```python
from build123d import *

# Parameters (mm, degrees)
BOSS_EXTRUDE1_DEPTH = 5
SKETCH2_R           = 2.5
BOSS_EXTRUDE2_DEPTH = 5
BOSS_EXTRUDE3_START = -2.644184
BOSS_EXTRUDE3_DEPTH = 127.644184


with BuildPart() as part:
    # Sketch1 → Boss-Extrude1 (new body)
    with BuildSketch(Plane(origin=(0, 0, 0), x_dir=(1, 0, 0), z_dir=(0, 1, 0))):
        with BuildLine():
            ThreePointArc((-22.5, 0), (0, -22.5), (22.5, 0))
            ThreePointArc((22.5, 0), (28.11402228, 25.340983158), (43.905514247, 45.939804848))
            ThreePointArc((43.905514247, 45.939804848), (54.788632448, 47.238126581), (60.325213459, 37.779047778))
            ThreePointArc((60.325213459, 37.779047778), (48.023832429, 20.66372887), (43.868302884, 0))
            ThreePointArc((43.868302884, 0), (0, -43.868302884), (-43.868302884, 0))
            ThreePointArc((-43.868302884, 0), (-48.023832429, 20.66372887), (-60.325213459, 37.779047778))
            ThreePointArc((-60.325213459, 37.779047778), (-54.788632448, 47.238126581), (-43.905514247, 45.939804848))
            ThreePointArc((-43.905514247, 45.939804848), (-28.11402228, 25.340983158), (-22.5, 0))
        make_face()
    extrude(amount=BOSS_EXTRUDE1_DEPTH)

    # Sketch2 → Boss-Extrude2 (add)
    with BuildSketch(Plane(origin=(0, 5, 0), x_dir=(1, 0, 0), z_dir=(0, 1, 0))):
        with Locations((28.779245994, -28.779245994)):
            Circle(SKETCH2_R)
        with Locations((-28.779245994, -28.779245994)):
            Circle(SKETCH2_R)
    extrude(amount=BOSS_EXTRUDE2_DEPTH)

    # Sketch4 → Boss-Extrude3 (add)
    with BuildSketch(Plane(origin=(0, 5, 43.868302884), x_dir=(1, 0, 0), z_dir=(0, 0, 1)).offset(BOSS_EXTRUDE3_START)):
        with BuildLine():
            Line((12.5, -5), (-12.5, -5))
            ThreePointArc((-12.5, -5), (-15, -2.5), (-12.5, 0))
            Line((-12.5, 0), (12.5, 0))
            ThreePointArc((12.5, 0), (15, -2.5), (12.5, -5))
        make_face()
    extrude(amount=BOSS_EXTRUDE3_DEPTH)


solid = part.part
```
Build history of the part. All positions in model axes, mm. A direction names the side the tool comes from. Round coordinates to 2 decimals unless told otherwise and drop trailing zeros. Write each loop counter-clockwise with the first axis right and the second up, starting at its lowest first coordinate (ties: lowest second). Pieces come first, ordered by that corner, then holes. Notation, with made-up numbers: (62.25, -38) -> (108.25, -38) arc R16 cw to (108.25, -30) -> close; hole circle Ø6 at (-10.5, 47.25). An arc over 180 degrees is marked (long way). Put each result on its own line as item: value.
Item 1: Two-plate mould, pull along X, no slides. Class faces 1 (the face through (15, 2.6, 104.2)), 2 (the face through (-28.27, 2.46, -25.67)), 3 (the face through (29, 10, 29)), 4 (the face through (-0.495, 2.465, 22.495)): pulls with the +X half, pulls with the -X half, needs draft (parallel to the pull), parting line crosses it, or undercut.
Here are the results:
face 1: pulls with the +X half
face 2: undercut
face 3: needs draft
face 4: undercut
Item 2: Tool access for faces 5 (the face through (27.96, 2.46, -25.01)), 6 (the face through (-15, 2.4, 104.2)), 7 (the face through (30.12, 7.46, 26.67)): list every direction of +Z, -Z, +X, -X, +Y, -Y with a clear straight run to the whole face (end or side of a thin tool).
Here are the results:
face 5: -Z, +Y, -Y
face 6: +Z, -X
face 7: +Y
Item 3: Slice it at A-A, the plane z = -22.5. Give the cut face in (x, y).
Here are the results:
outline: (-48.87, 0) -> (-26.88, 0) -> (-26.88, 5) -> (-48.87, 5) -> close; (26.88, 0) -> (48.87, 0) -> (48.87, 5) -> (26.88, 5) -> close
Item 4: Slice it at B-B, the plane y = 2.5. Give the cut face in (x, z), plus the area to 3 significant figures.
Here are the results:
outline: (-60.33, -37.78) arc R10 ccw to (-43.91, -45.94) arc R60 ccw to (-22.5, 0) arc R22.5 cw to (22.5, 0) arc R60 ccw to (43.91, -45.94) arc R10 ccw to (60.33, -37.78) arc R50 cw to (43.87, 0) arc R43.87 ccw to (15, 41.22) -> (15, 168.87) -> (-15, 168.87) -> (-15, 41.22) arc R43.87 ccw to (-43.87, 0) arc R50 cw to start
area: 8,040 mm^2
Item 5: Slice it at C-C, the plane x = 0. Give the cut face in (y, z), plus the area to 3 significant figures.
Here are the results:
outline: (0, 22.5) -> (5, 22.5) -> (5, 168.87) -> (0, 168.87) -> close
area: 732 mm^2
Item 6: Wall check: probe 1 along X at (y, z) = (4.5, 1); probe 2 along X at (y, z) = (2, 122); probe 3 along Z at (x, y) = (28.5, 7). Give the ranges that are in metal, low to high. Write a range as from..to.
Here are the results:
probe 1: x = -43.86..-22.48, 22.48..43.86
probe 2: x = -14.95..14.95
probe 3: z = 26.29..31.26
Item 7: Flat gauge pins, fed straight in: P1, Ø4, axis at y = 3.5, z = 88, coming from the +X side; P2, Ø5, axis at x = 36, y = 2.5, coming from the +Z side; P3, Ø1, axis at x = -38, y = 6, coming from the -Z side; P4, Ø1.5, axis at y = 2.5, z = 103, coming from the -X side. Where does each tip first touch, or does it go through?
Here are the results:
P1: stops at x = 15
P2: stops at z = 28.32
P3: passes through
P4: stops at x = -15
Item 8: Slice it at D-D, the plane z = 19. Give the cut face in (x, y), plus the area to 3 significant figures.
Here are the results:
outline: (-39.54, 0) -> (-12.05, 0) -> (-12.05, 5) -> (-39.54, 5) -> close; (12.05, 0) -> (39.54, 0) -> (39.54, 5) -> (12.05, 5) -> close
area: 275 mm^2
